from build123d import *

# Parameters (mm, degrees)
SKETCH1_R           = 2.1
BOSS_EXTRUDE1_DEPTH = 156.74
CUT_EXTRUDE1_DEPTH  = 159.326964223


with BuildPart() as part:
    # Sketch1 → Boss-Extrude1 (new body)
    with BuildSketch(Plane.XY):
        with BuildLine():
            Line((-4.9, -10), (-3.1, -8.2))
            Line((-3.1, -8.2), (-5.5, -8.2))
            Line((-5.5, -8.2), (-5.5, -6.560660172))
            Line((-5.5, -6.560660172), (-2.539339828, -3.6))
            Line((-2.539339828, -3.6), (2.539339828, -3.6))
            Line((2.539339828, -3.6), (5.5, -6.560660172))
            Line((5.5, -6.560660172), (5.5, -8.2))
            Line((5.5, -8.2), (3.1, -8.2))
            Line((3.1, -8.2), (4.9, -10))
            Line((4.9, -10), (8, -10))
            ThreePointArc((8, -10), (9.414213562, -9.414213562), (10, -8))
            Line((10, -8), (10, -4.9))
            Line((10, -4.9), (8.2, -3.1))
            Line((8.2, -3.1), (8.2, -5.5))
            Line((8.2, -5.5), (6.560660172, -5.5))
            Line((6.560660172, -5.5), (3.6, -2.539339828))
            Line((3.6, -2.539339828), (3.6, 2.539339828))
            Line((3.6, 2.539339828), (6.560660172, 5.5))
            Line((6.560660172, 5.5), (8.2, 5.5))
            Line((8.2, 5.5), (8.2, 3.1))
            Line((8.2, 3.1), (10, 4.9))
            Line((10, 4.9), (10, 8))
            ThreePointArc((10, 8), (9.414213562, 9.414213562), (8, 10))
            Line((8, 10), (4.9, 10))
            Line((4.9, 10), (3.1, 8.2))
            Line((3.1, 8.2), (5.5, 8.2))
            Line((5.5, 8.2), (5.5, 6.560660172))
            Line((5.5, 6.560660172), (2.539339828, 3.6))
            Line((2.539339828, 3.6), (-2.539339828, 3.6))
            Line((-2.539339828, 3.6), (-5.5, 6.560660172))
            Line((-5.5, 6.560660172), (-5.5, 8.2))
            Line((-5.5, 8.2), (-3.1, 8.2))
            Line((-3.1, 8.2), (-4.9, 10))
            Line((-4.9, 10), (-8, 10))
            ThreePointArc((-8, 10), (-9.414213562, 9.414213562), (-10, 8))
            Line((-10, 8), (-10, 4.9))
            Line((-10, 4.9), (-8.2, 3.1))
            Line((-8.2, 3.1), (-8.2, 5.5))
            Line((-8.2, 5.5), (-6.560660172, 5.5))
            Line((-6.560660172, 5.5), (-3.6, 2.539339828))
            Line((-3.6, 2.539339828), (-3.6, -2.539339828))
            Line((-3.6, -2.539339828), (-6.560660172, -5.5))
            Line((-6.560660172, -5.5), (-8.2, -5.5))
            Line((-8.2, -5.5), (-8.2, -3.1))
            Line((-8.2, -3.1), (-10, -4.9))
            Line((-10, -4.9), (-10, -8))
            ThreePointArc((-10, -8), (-9.414213562, -9.414213562), (-8, -10))
            Line((-8, -10), (-4.9, -10))
        make_face()
        Circle(SKETCH1_R, mode=Mode.SUBTRACT)
    extrude(amount=BOSS_EXTRUDE1_DEPTH)

    # Sketch2 → Cut-Extrude1 (cut, through all)
    with BuildSketch(Plane(origin=(10, 0, 0), x_dir=(0, 0, -1), z_dir=(1, 0, 0))):
        Polygon((-156.74, 10), (-136.74, -10), (-156.74, -10), align=None)
        Polygon((0, 10), (-20, -10), (0, -10), align=None)
    extrude(amount=-CUT_EXTRUDE1_DEPTH, mode=Mode.SUBTRACT)


solid = part.part
Work out the finished part from the listing and answer in its coordinate system (mm). A direction names the side the tool comes from. Coordinates: 2 decimals unless noted, no trailing zeros. Loops run counter-clockwise (first coordinate to the right, second up) from the corner with the lowest first, then second, coordinate; pieces in that order, holes last. Notation, with made-up numbers: M 40.5,25.25 L 74.5,25.25 A11 ccw 74.5,39.25 Z; hole C 58.5,62 d3. An arc over 180 degrees is marked long. Answer in a Markdown table with one row per item. Add a question column.
1. Flat-ended cylindrical pins translate along their axes: P1, Ø3, axis at x = 4, y = 5.5, coming from the +Z side; P2, Ø3, axis at x = 5.5, y = -7.5, coming from the +Z side; P3, Ø1.5, axis at x = 1, z = 90.5, coming from the +Y side. Find the tip coordinate at first contact, or state that the pin passes through.
2. Consider L1, parallel to Y at x = 0, z = 67.5; L2, parallel to X at y = -7.75, z = 120.5; L3, parallel to Y at x = 5, z = 119.5. Determine where each line is inside the solid, lowest interval first.
3. Find section B-B, the plane x = 0. Write down the section's boundary in (y, z).
4. A tool of negligible diameter and unlimited length cuts with its end or side. For faces 5 (the flat face through (0, -3.6, 77)), 6 (the flat face through (-3.6, 0, 77)), 7 (the flat face through (-5.1, 4.04, 77.34)), from which of +Z, -Z, +X, -X, +Y, -Y can it reach the whole face along a straight path? Write none if from no direction.
5. Find section A-A, the plane y = 0. Write down the section's boundary in (x, z), then the cut area to 3 significant figures.
6. The mould has two halves that part along X. Classify faces 1 (the flat face through (6, -10, 78)), 2 (the flat face through (-4, -8.2, 78)), 3 (the flat face through (-10, -6, 77)), 4 (the flat face through (10, -6, 77)): pulls with the +X half, pulls with the -X half, needs draft (parallel to the pull), parting line crosses it, or undercut.
Reported:
| question | item | result |
|---|---|---|
| 1 | P1 | stops at z = 153.06 |
| 1 | P2 | stops at z = 140.74 |
| 1 | P3 | stops at y = 3.6 |
| 2 | L1 | y = -3.6 to -2.1, 2.1 to 3.6 |
| 2 | L2 | x = -10 to -5.5, 5.5 to 10 |
| 2 | L3 | y = -10 to -8.2, -6.06 to -3.94, 3.94 to 6.06, 8.2 to 10 |
| 3 | outline | M -3.6,13.6 L -2.1,12.1 L -2.1,144.64 L -3.6,143.14 Z; M 2.1,7.9 L 3.6,6.4 L 3.6,150.34 L 2.1,148.84 Z |
| 4 | face 5 | +Z, -Z, -Y |
| 4 | face 6 | +Z, -Z, -X |
| 4 | face 7 | +Z, -Z |
| 5 | outline | M -3.6,10 L -2.1,10 L -2.1,146.74 L -3.6,146.74 Z; M 2.1,10 L 3.6,10 L 3.6,146.74 L 2.1,146.74 Z |
| 5 | area | 410 mm^2 |
| 6 | face 1 | needs draft |
| 6 | face 2 | undercut |
| 6 | face 3 | pulls with the -X half |
| 6 | face 4 | pulls with the +X half |
